The model under review builds one solid part; all positions refer to its coordinate system, in mm. Face numbers are marked on the shaded views. A direction names the side the tool comes from. Coordinates: 2 decimals unless noted, no trailing zeros. Write each loop counter-clockwise with the first axis right and the second up, starting at its lowest first coordinate (ties: lowest second). Pieces come first, ordered by that corner, then holes. Notation, with made-up numbers: (18.5, -11.75) - (76.5, -11.75) arc R22 cw to (76.5, 7.25) - close; hole circle Ø5 at (47, 45.5). An arc over 180 degrees is marked (long way). Put each result on its own line as item: value.
Autodesk Inventor part; units mm, degrees
ref_plane "YZ Plane" through (0, 0, 0) normal (1, 0, 0) x (0, 1, 0)
ref_plane "XZ Plane" through (0, 0, 0) normal (0, 1, 0) x (-1, 0, 0)
ref_plane "XY Plane" through (0, 0, 0) normal (0, 0, 1) x (1, 0, 0)
sketch "Sketch1" plane through (0, 0, 0) normal (0, 1, 0) x (-1, 0, 0)
  line L0 (0, 0) -> (5.588, 0)
  line L1 (5.588, 0) -> (5.588, -5.588)
  line L2 (5.588, -5.588) -> (0, -5.588)
  line L3 (0, -5.588) -> (0, 0)
  dimension "d0" = 5.588
  dimension "d1" = 5.588
extrude "Extrusion1" add sketch "Sketch1" along normal blind 5.588
chamfer "Chamfer1" distance 1.016 distance2 3.175 1 edges at (-2.794, 5.588, 0) measured on face at (-1.8627, 5.588, -1.8627)
sketch "Sketch2" plane through (0, 5.588, 0) normal (0, 1, 0) x (1, 0, 0)
  line L0 (0, 1.016) -> (-5.588, 1.016)
  line L1 (0, 1.016) -> (0, 5.588)
  line L2 (0, 5.588) -> (-5.588, 5.588)
  line L3 (-5.588, 5.588) -> (-5.588, 1.016)
  circle A0 centre (-4.064, 3.302) radius 0.9525
  circle A1 centre (-1.524, 3.302) radius 0.9525
  point P0 (0, 0)
  dimension "d7" = 1.905
  dimension "d8" = 1.905
  dimension "d9" = 1.524
  dimension "d10" = 1.524
extrude "Extrusion2" cut sketch "Sketch2" against normal blind 2.54 contours A0 | A1
properties part number "connector"
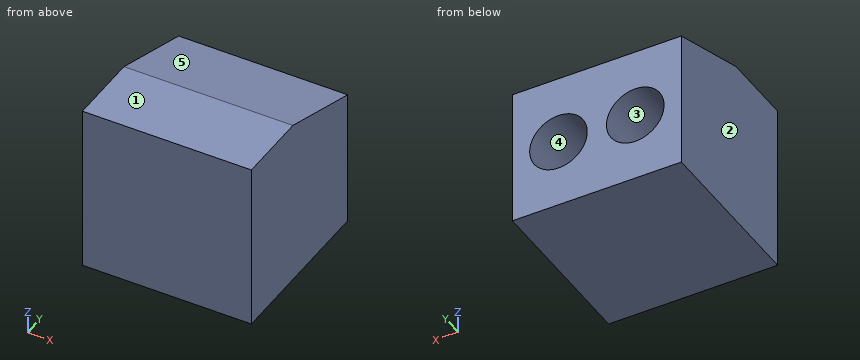
1. Machinability: for the marked faces 4 and 5, which of the approach directions +Z, -Z, +X, -X, +Y, -Y give a long, thin tool a straight path to every point of the face, cutting with its end or side? Answer none if there is none.
Determined:
face 4: +Y
face 5: +Z, +X, -X, +Y
2. Consider section A-A on x = -4.3. State the section outline as (y, z) points, plus the area to 3 significant figures.
Determined:
outline: (0, -5.59) - (5.59, -5.59) - (5.59, -4.22) - (3.05, -4.22) - (3.05, -2.38) - (5.59, -2.38) - (5.59, -1.02) - (2.41, 0) - (0, 0) - close
area: 24.9 mm^2
3. To check wall thickness, follow probe 1 along X at (y, z) = (5.3, -3.55); probe 2 along X at (y, z) = (4.7, -2.8); probe 3 along Y at (x, z) = (-4.4, -3.1). State the ranges of each line that lie inside material, in increasing order.
Determined:
probe 1: x = -5.59 to -4.98, -3.14 to -2.44, -0.6 to 0
probe 2: x = -5.59 to -4.87, -3.25 to -2.33, -0.71 to 0
probe 3: y = 0 to 3.05
4. For pin 1 Ø1.5 at (x, z) = (-1.524, -3.302) entering from +Y, flat-tipped, find the tip position at first contact; note if it passes through.
Determined:
pin 1: stops at y = 3.05
5. Consider section D-D on x = -1.7. State the section outline as (y, z) points.
Determined:
outline: (0, -5.59) - (5.59, -5.59) - (5.59, -4.24) - (3.05, -4.24) - (3.05, -2.37) - (5.59, -2.37) - (5.59, -1.02) - (2.41, 0) - (0, 0) - close
6. Consider section B-B on y = 3.55. State the section outline as (x, z) points (1 decimal), plus the area to 3 significant figures.
Determined:
outline: (-5.6, -5.6) - (0, -5.6) - (0, -0.4) - (-5.6, -0.4) - close; hole circle Ø1.9 at (-4.1, -3.3); hole circle Ø1.9 at (-1.5, -3.3)
area: 23.5 mm^2
7. The part is to be moulded in two halves that separate along Z. For the marked faces 1, 2 and 3, say which applies: +Z half, -Z half, draft (parallel to the pull), parting line (faces both ways), or undercut.
Determined:
face 1: +Z half
face 2: draft
face 3: undercut
8. Consider section C-C on z = -2.5. State the section outline as (x, y) points.
Determined:
outline: (-5.59, 0) - (0, 0) - (0, 5.59) - (-1.01, 5.59) - (-1.01, 3.05) - (-2.04, 3.05) - (-2.04, 5.59) - (-3.55, 5.59) - (-3.55, 3.05) - (-4.58, 3.05) - (-4.58, 5.59) - (-5.59, 5.59) - close
